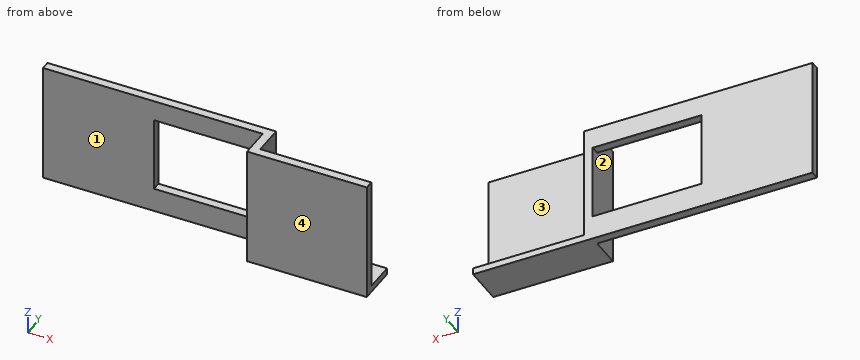
Autodesk Inventor part; units mm, degrees
ref_plane "YZ Plane" through (0, 0, 0) normal (1, 0, 0) x (0, 1, 0)
ref_plane "XZ Plane" through (0, 0, 0) normal (0, 1, 0) x (-1, 0, 0)
ref_plane "XY Plane" through (0, 0, 0) normal (0, 0, 1) x (1, 0, 0)
sketch "Sketch1" plane through (0, 0, 0) normal (0, 1, 0) x (-1, 0, 0)
  line L0 (71.974, 9.2811) -> (-6.026, 9.2811)
  line L1 (-6.026, 9.2811) -> (-6.026, -18.2189)
  line L2 (-6.026, -18.2189) -> (71.974, -18.2189)
  line L3 (71.974, -18.2189) -> (71.974, 9.2811)
  point P0 (0, 0)
  dimension "d0" = 27.5
  dimension "d1" = 78
extrude "Extrusion1" add sketch "Sketch1" along normal blind 9
sketch "Sketch2" plane through (0, 9, 0) normal (0, 1, 0) x (1, 0, 0)
  line L0 (6.026, 18.2189) -> (-71.974, 18.2189)
  line L1 (-71.974, -9.2811) -> (6.026, -9.2811)
  line L2 (6.026, 18.2189) -> (-19.474, 18.2189)
  line L3 (-19.474, 18.2189) -> (-19.474, -9.2811)
  line L4 (-19.474, -9.2811) -> (6.026, -9.2811)
  line L5 (6.026, -9.2811) -> (6.026, 18.2189)
  point P0 (0, 0)
  point P1 (6.026, -9.2811)
  point P2 (-19.474, 18.2189)
  dimension "d4" = 25.5
extrude "Extrusion2" cut sketch "Sketch2" against normal blind 7
sketch "Sketch3" plane through (0, 2, 0) normal (0, 1, 0) x (1, 0, 0)
  point P0 (0, 0)
sketch "Sketch4" plane through (0, 2, 0) normal (0, 1, 0) x (1, 0, 0)
  line L0 (-19.474, -9.2811) -> (-19.474, 18.2189)
  line L1 (6.026, -9.2811) -> (6.026, 18.2189)
  line L2 (-19.474, 18.2189) -> (6.026, 18.2189)
  line L3 (6.026, 18.2189) -> (6.026, 16.7189)
  line L4 (6.026, 16.7189) -> (-19.474, 16.7189)
  line L5 (-19.474, 16.7189) -> (-19.474, 18.2189)
  point P0 (0, 0)
  point P1 (6.026, 18.2189)
  point P2 (-19.474, 16.7189)
  dimension "d7" = 1.5
extrude "Extrusion3" add sketch "Sketch4" along normal blind 7
sketch "Sketch5" plane through (-71.974, 0, 9.2811) normal (0, 0, 1) x (1, 0, 0)
  line L0 (0, 9) -> (52.5, 9)
  line L1 (50.5, 9) -> (50.5, 0)
  line L2 (0, 0) -> (78, 0)
  line L3 (52.5, 2) -> (52.5, 9)
  line L4 (50.5, 7) -> (0, 7)
  line L5 (52.5, 2) -> (52.5, 9)
  line L6 (0, 9) -> (52.5, 9)
  line L7 (0, 0) -> (0, 9)
  line L8 (0, 0) -> (78, 0)
  line L9 (78, 0) -> (78, 2)
  line L10 (78, 2) -> (52.5, 2)
  point P0 (71.974, 0)
  point P1 (0, 7)
  dimension "d10" = 2
  dimension "d11" = 2
extrude "Extrusion4" cut sketch "Sketch5" against normal blind 44 contours L4 L1 L2 L7
sketch "Sketch8" plane through (-71.974, 7, 9.2811) normal (0, -1, 0) x (1, 0, 0)
  line L0 (50.5, -21.9505) -> (25.5, -21.9505)
  line L1 (25.5, -21.9505) -> (25.5, -4.7505)
  line L2 (25.5, -4.7505) -> (50.5, -4.7505)
  line L3 (50.5, -4.7505) -> (50.5, -21.9505)
  line L4 (50.5, 0) -> (50.5, -27.5)
  point P0 (71.974, -9.2811)
  dimension "d20" = 17.2
  dimension "d21" = 25
  dimension "d22" = 0
extrude "Extrusion6" cut sketch "Sketch8" against normal blind 2
ref_plane "Work Plane1" through (-20.474, 2, 9.2811) normal (1, 0, 0) x (0, 0, -1)
sketch "Sketch10" plane through (0, 9, 0) normal (0, 1, 0) x (1, 0, 0)
  point P0 (0, 0)
properties part number "gps _mount"
The listing builds one solid part. Answer for the finished solid, in the listing's coordinates (mm). Face numbers are marked on the shaded views. A direction names the side the tool comes from. Round coordinates to 2 decimals unless told otherwise and drop trailing zeros. Order: outer loops, then holes, each group sorted by start corner. A loop starts at its lowest first (then second) coordinate and runs counter-clockwise, first axis right, second up. Notation, with made-up numbers: M -40,10 L -15,10 A34 ccw -15,48 Z; hole C -17,34 d9. An arc over 180 degrees is marked long. Answer in a Markdown table with one row per item. Add a question column.
1) Consider line 1 along X through (y, z) = (8.25, -7); line 2 along Z through (x, y) = (-8, 8); line 3 along Y through (x, z) = (-7.5, -6). Determine where each line is inside the solid, lowest interval first. Write a range as from..to.
2) Flat-ended cylindrical pins translate along their axes: pin 1 Ø8 at (x, z) = (-39.5, -5.5) entering from -Y; pin 2 Ø12 at (x, z) = (-60, -4) entering from -Y; pin 3 Ø3.5 at (y, z) = (6.5, -5) entering from +X; pin 4 Ø7.5 at (x, z) = (-7, -8) entering from +Y. Find the tip coordinate at first contact, or state that the pin passes through.
3) The part is cut by section D-D on z = 5.75. Determine the outline of the cut face in (x, y).
4) The part is cut by section B-B on z = -5.5. Determine the outline of the cut face in (x, y).
5) The part is cut by section C-C on y = 8. Determine the outline of the cut face in (x, z), plus the area to 3 significant figures.
6) Determine the mould class of the marked faces 1 and 2 for opening direction X: pulls with the +X half, pulls with the -X half, needs draft (parallel to the pull), parting line crosses it, or undercut.
7) Which of the six approach directions +Z, -Z, +X, -X, +Y, -Y give full straight-line access (tool end or side, diameter ignored) to the marked faces 3 and 4?
8) The part is cut by section A-A on x = -28. Determine the outline of the cut face in (y, z).
Findings below:
| question | item | result |
|---|---|---|
| 1 | line 1 | x = -71.97..-46.47, -21.47..-19.47 |
| 1 | line 2 | z = -18.22..-16.72 |
| 1 | line 3 | y = 0..2 |
| 2 | pin 1 | passes through |
| 2 | pin 2 | stops at y = 7 |
| 2 | pin 3 | stops at x = -19.47 |
| 2 | pin 4 | stops at y = 2 |
| 3 | outline | M -71.97,7 L -21.47,7 L -21.47,0 L 6.03,0 L 6.03,2 L -19.47,2 L -19.47,9 L -71.97,9 Z |
| 4 | outline | M -71.97,7 L -46.47,7 L -46.47,9 L -71.97,9 Z; M -21.47,0 L 6.03,0 L 6.03,2 L -19.47,2 L -19.47,9 L -21.47,9 Z |
| 5 | outline | M -71.97,-18.22 L 6.03,-18.22 L 6.03,-16.72 L -19.47,-16.72 L -19.47,9.28 L -71.97,9.28 Z; hole M -46.47,-12.67 L -21.47,-12.67 L -21.47,4.53 L -46.47,4.53 Z |
| 5 | area | 1,050 mm² |
| 6 | face 1 | needs draft |
| 6 | face 2 | undercut |
| 7 | face 3 | +Z, +X, +Y |
| 7 | face 4 | +Z, -Z, +X, -X, -Y |
| 8 | outline | M 7,-18.22 L 9,-18.22 L 9,-12.67 L 7,-12.67 Z; M 7,4.53 L 9,4.53 L 9,9.28 L 7,9.28 Z |
